Input: part model. Units: mm. Frame: model coordinates. Face numbers are marked on the shaded views. Coordinates: 2 decimals unless noted, no trailing zeros. Order: outer loops, then holes, each group sorted by start corner. A loop starts at its lowest first (then second) coordinate and runs counter-clockwise, first axis right, second up. Notation, with made-up numbers: (36.5, -22) - (66.5, -22) arc R7 ccw to (66.5, -15) - close; hole circle Ø1 at (51, -40). An arc over 180 degrees is marked (long way). One line per question, with ' | ' between items.
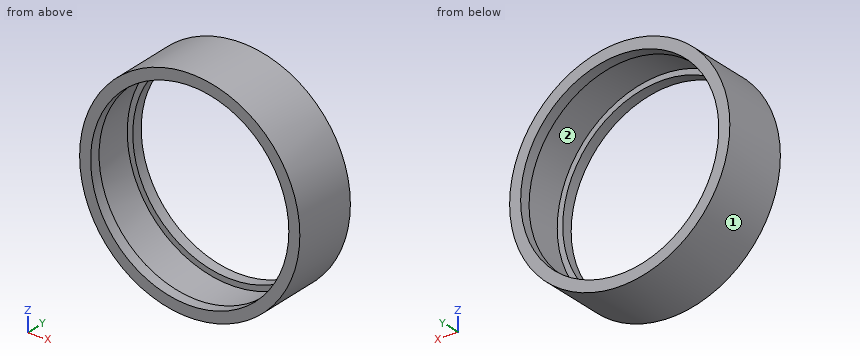
Autodesk Inventor part; units mm, degrees
ref_plane "YZ Plane" through (0, 0, 0) normal (1, 0, 0) x (0, 1, 0)
ref_plane "XZ Plane" through (0, 0, 0) normal (0, 1, 0) x (-1, 0, 0)
ref_plane "XY Plane" through (0, 0, 0) normal (0, 0, 1) x (1, 0, 0)
sketch "Sketch1" plane through (0, 0, 0) normal (0, 0, 1) x (1, 0, 0)
  line L0 (-1.7455, 0) -> (-1.7455, 9.9919)
  line L1 (2.7545, 5.5444) -> (2.7545, 6.0444)
  line L2 (2.7545, 6.0444) -> (3.2545, 6.0444)
  line L3 (3.2545, 6.0444) -> (3.2545, 3.0444)
  line L4 (3.2545, 3.0444) -> (2.7545, 3.0444)
  line L5 (2.7545, 3.0444) -> (2.7545, 3.5444)
  line L6 (2.7545, 5.5444) -> (3.0045, 5.5444)
  line L7 (3.0045, 5.5444) -> (3.0045, 3.5444)
  line L8 (3.0045, 3.5444) -> (2.7545, 3.5444)
  dimension "d5" = 3
  dimension "d13" = 0.25
  dimension "d14" = 10
  dimension "d15" = 0.5
  dimension "d16" = 9.5
revolve "Revolution1" add sketch "Sketch1" angle 360 about axis through (-1.7455, 0, 0) along (0, 1, 0)
properties part number "Out"
Item 1: Section B-B on x = 1.5. Return the cut outline in (y, z).
Data:
outline: (3.04, -3.8) - (6.04, -3.8) - (6.04, -3.12) - (5.54, -3.12) - (5.54, -3.47) - (3.54, -3.47) - (3.54, -3.12) - (3.04, -3.12) - close; (3.04, 3.12) - (3.54, 3.12) - (3.54, 3.47) - (5.54, 3.47) - (5.54, 3.12) - (6.04, 3.12) - (6.04, 3.8) - (3.04, 3.8) - close
Item 2: Contact query for flat-ended pins moving along their axis: P1, Ø5.5, axis at x = -1.75, z = 0, coming from the -Y side; P2, Ø1.5, axis at y = 4, z = 1, coming from the +X side. Output: stop coordinate, or through.
Data:
P1: through | P2: x = 3.25
Item 3: Draft query along X for the marked faces 1 and 2. Return one class per face: released by +X, released by -X, zero draft, split by the parting line, or undercut.
Data:
face 1: split by the parting line | face 2: undercut
Item 4: Section A-A on z = 0. Return the cut outline in (x, y), and give its area (3 significant figures).
Data:
outline: (-6.75, 3.04) - (-6.25, 3.04) - (-6.25, 3.54) - (-6.5, 3.54) - (-6.5, 5.54) - (-6.25, 5.54) - (-6.25, 6.04) - (-6.75, 6.04) - close; (2.75, 3.04) - (3.25, 3.04) - (3.25, 6.04) - (2.75, 6.04) - (2.75, 5.54) - (3, 5.54) - (3, 3.54) - (2.75, 3.54) - close | area: 2.00 mm^2
Item 5: Section C-C on y = 4.6. Return the cut outline in (x, z).
Data:
outline: circle Ø10 at (-1.75, 0); hole circle Ø9.5 at (-1.75, 0)
Item 6: Ray query, line 1 (X direction, y = 3.35, z = 0); line 2 (Y direction, x = 0.5, z = 4); line 3 (Z direction, x = -6, y = 5.3). Return the intervals inside material, ascending.
Data:
line 1: -6.75 to -6.25, 2.75 to 3.25 | line 2: 3.04 to 3.54, 5.54 to 6.04 | line 3: -2.63 to -2.11, 2.11 to 2.63
